```python
from build123d import *

# Parameters (mm, degrees)
SKETCH2_R           = 4
BOSS_EXTRUDE1_DEPTH = 40


with BuildPart() as part:
    # Sketch2 → Boss-Extrude1 (new body)
    with BuildSketch(Plane.XY):
        with BuildLine():
            Line((25, 7.5), (0, 7.5))
            ThreePointArc((0, 7.5), (-7.5, 0), (0, -7.5))
            Line((0, -7.5), (25, -7.5))
            ThreePointArc((25, -7.5), (27.255293496, -7.152877131), (29.301823273, -6.143640332))
            Line((29.301823273, -6.143640332), (90.166313701, 36.474134675))
            Line((90.166313701, 36.474134675), (87.585219737, 40.160318874))
            Line((87.585219737, 40.160318874), (72.510818569, 40.767433308))
            Line((72.510818569, 40.767433308), (25, 7.5))
        make_face()
        Circle(SKETCH2_R, mode=Mode.SUBTRACT)
        with Locations((25, 0)):
            Circle(SKETCH2_R, mode=Mode.SUBTRACT)
    extrude(amount=BOSS_EXTRUDE1_DEPTH)


solid = part.part
```
The model under review builds one solid part; all positions refer to its coordinate system, in mm. Round coordinates to 2 decimals unless told otherwise and drop trailing zeros. Order: outer loops, then holes, each group sorted by start corner. A loop starts at its lowest first (then second) coordinate and runs counter-clockwise, first axis right, second up.
Item 1: Draft analysis for pull direction Y (two halves, no side actions). For faces 1 (the flat face through (59.31, 14.87, 19.72)), 2 (the flat face through (13, 7.5, 20)), 3 (the cylindrical face through (-0.867, -3.905, 19.72)), state which applies: released by +Y, released by -Y, zero draft, split by the parting line, or undercut.
Working result:
face 1: released by -Y
face 2: released by +Y
face 3: undercut
Item 2: To check wall thickness, follow probe 1 along Y at (x, z) = (0, 17.5); probe 2 along X at (y, z) = (-1, 23); probe 3 along X at (y, z) = (2.5, 30). State the ranges of each line that lie inside material, in increasing order.
Working result:
probe 1: y = -7.5 to -4, 4 to 7.5
probe 2: x = -7.43 to -3.87, 3.87 to 21.13, 28.87 to 36.65
probe 3: x = -7.07 to -3.12, 3.12 to 21.88, 28.12 to 41.65
Item 3: Add section A-A, the plane z = 17. State the section outline as (x, y) points, and give its area (3 significant figures).
Working result:
outline: (0, -7.5) - (25, -7.5) arc R7.5 ccw to (29.3, -6.14) - (90.17, 36.47) - (87.59, 40.16) - (72.51, 40.77) - (25, 7.5) - (0, 7.5) arc R7.5 ccw to start; hole circle Ø8 at (0, 0); hole circle Ø8 at (25, 0)
area: 1,330 mm2
Item 4: Add section B-B, the plane y = -3. State the section outline as (x, z) points, and give its area (3 significant figures).
Working result:
outline: (-6.87, 0) - (-2.65, 0) - (-2.65, 40) - (-6.87, 40) - close; (2.65, 0) - (22.35, 0) - (22.35, 40) - (2.65, 40) - close; (27.65, 0) - (33.79, 0) - (33.79, 40) - (27.65, 40) - close
area: 1,200 mm2
Item 5: Add section D-D, the plane y = 17. State the section outline as (x, z) points.
Working result:
outline: (38.57, 0) - (62.35, 0) - (62.35, 40) - (38.57, 40) - close
Item 6: For pin 1 (1.5 mm diameter, centred on x = 38, z = 6, fed in from +Y); pin 2 (20 mm diameter, centred on x = 14.5, z = 19, fed in from +Y); pin 3 (3 mm diameter, centred on y = 30, z = 14.5, fed in from +X), all flat-tipped, find the tip position at first contact; note any pin that passes through.
Working result:
pin 1: stops at y = 17.13
pin 2: stops at y = 7.5
pin 3: stops at x = 83.06
Item 7: Add section C-C, the plane x = 18. State the section outline as (y, z) points, and give its area (3 significant figures).
Working result:
outline: (-7.5, 0) - (7.5, 0) - (7.5, 40) - (-7.5, 40) - close
area: 600 mm2
